The model under review builds one solid part; all positions refer to its coordinate system, in mm. Face numbers are marked on the shaded views. A direction names the side the tool comes from. Coordinates: 2 decimals unless noted, no trailing zeros. Write each loop counter-clockwise with the first axis right and the second up, starting at its lowest first coordinate (ties: lowest second). Pieces come first, ordered by that corner, then holes.
Autodesk Inventor part; units mm, degrees
ref_plane "YZ Plane" through (0, 0, 0) normal (1, 0, 0) x (0, 1, 0)
ref_plane "XZ Plane" through (0, 0, 0) normal (0, 1, 0) x (-1, 0, 0)
ref_plane "XY Plane" through (0, 0, 0) normal (0, 0, 1) x (1, 0, 0)
sketch "Sketch1" plane through (0, 0, 0) normal (0, 1, 0) x (-1, 0, 0)
  arc A0 (52.0258, 55.1946) -> (51.0258, 56.1946) centre (51.0258, 55.1946) ccw
  line L0 (-43.9742, 56.1946) -> (51.0258, 56.1946)
  arc A1 (-43.9742, 56.1946) -> (-44.9742, 55.1946) centre (-43.9742, 55.1946) ccw
  line L1 (-44.9742, -39.8054) -> (-44.9742, 55.1946)
  arc A2 (-44.9742, -39.8054) -> (-43.9742, -40.8054) centre (-43.9742, -39.8054) ccw
  line L2 (51.0258, -40.8054) -> (-43.9742, -40.8054)
  arc A3 (51.0258, -40.8054) -> (52.0258, -39.8054) centre (51.0258, -39.8054) ccw
  line L3 (52.0258, 55.1946) -> (52.0258, -39.8054)
  line L4 (-11.2742, 54.1946) -> (-42.9742, 54.1946)
  line L5 (-11.2742, -38.8054) -> (-11.2742, 54.1946)
  line L6 (-42.9742, -38.8054) -> (-11.2742, -38.8054)
  line L7 (-42.9742, 54.1946) -> (-42.9742, -38.8054)
  line L8 (50.0258, -38.8054) -> (50.0258, 54.1946)
  line L9 (-9.2742, -38.8054) -> (50.0258, -38.8054)
  line L10 (-9.2742, 54.1946) -> (-9.2742, -38.8054)
  line L11 (50.0258, 54.1946) -> (-9.2742, 54.1946)
  line L12 (53.5258, 57.6946) -> (-46.4742, 57.6946)
  line L13 (-46.4742, 57.6946) -> (-46.4742, -42.3054)
  line L14 (-46.4742, -42.3054) -> (53.5258, -42.3054)
  line L15 (53.5258, -42.3054) -> (53.5258, 57.6946)
  line L16 (51.0258, 55.1946) -> (-43.9742, 55.1946) construction
  line L17 (-43.9742, 55.1946) -> (-43.9742, -39.8054) construction
  line L18 (-43.9742, -39.8054) -> (51.0258, -39.8054) construction
  line L19 (51.0258, -39.8054) -> (51.0258, 55.1946) construction
  line L20 (-41.4742, -37.3054) -> (-12.7742, -37.3054)
  line L21 (-12.7742, -37.3054) -> (-12.7742, 52.6946)
  line L22 (-12.7742, 52.6946) -> (-41.4742, 52.6946)
  line L23 (-41.4742, 52.6946) -> (-41.4742, -37.3054)
  line L24 (-7.7742, -37.3054) -> (48.5258, -37.3054)
  line L25 (48.5258, -37.3054) -> (48.5258, 52.6946)
  line L26 (48.5258, 52.6946) -> (-7.7742, 52.6946)
  line L27 (-7.7742, 52.6946) -> (-7.7742, -37.3054)
  line L28 (-10.2742, 55.1946) -> (-10.2742, -39.8054) construction
  arc A4 (51.0258, -40.6054) -> (51.8258, -39.8054) centre (51.0258, -39.8054) ccw
  line L29 (51.0258, -40.6054) -> (-43.9742, -40.6054)
  arc A5 (-44.7742, -39.8054) -> (-43.9742, -40.6054) centre (-43.9742, -39.8054) ccw
  line L30 (-44.7742, -39.8054) -> (-44.7742, 55.1946)
  arc A6 (-43.9742, 55.9946) -> (-44.7742, 55.1946) centre (-43.9742, 55.1946) ccw
  line L31 (-43.9742, 55.9946) -> (51.0258, 55.9946)
  arc A7 (51.8258, 55.1946) -> (51.0258, 55.9946) centre (51.0258, 55.1946) ccw
  line L32 (51.8258, 55.1946) -> (51.8258, -39.8054)
  line L33 (50.2258, 54.3946) -> (50.2258, -39.0054)
  line L34 (50.2258, -39.0054) -> (-9.4742, -39.0054)
  line L35 (-9.4742, -39.0054) -> (-9.4742, 54.3946)
  line L36 (-9.4742, 54.3946) -> (50.2258, 54.3946)
  line L37 (-43.1742, -39.0054) -> (-11.0742, -39.0054)
  line L38 (-11.0742, -39.0054) -> (-11.0742, 54.3946)
  line L39 (-11.0742, 54.3946) -> (-43.1742, 54.3946)
  line L40 (-43.1742, 54.3946) -> (-43.1742, -39.0054)
  point P0 (0, 0)
  point P1 (-29.6242, 39.9946)
  dimension "d0" = 2
  dimension "d1" = 2.5
  dimension "d2" = 2.5
  dimension "d3" = 2.5
  dimension "d4" = 2.5
  dimension "d5" = 2.5
  dimension "d6" = 2.5
  dimension "d7" = 2.5
  dimension "d8" = 2.5
  dimension "d9" = 5
  dimension "d10" = 1
  dimension "d11" = 2
  dimension "d12" = 2.5
  dimension "d13" = 0.2
  dimension "d14" = 0.2
  dimension "d15" = 0.2
extrude "Extrusion1" add sketch "Sketch1" along normal blind 5 contours L3 A3 L2 A2 L1 A1 L0 A0 | L5 L6 L7 L4 | L9 L10 L11 L8 | L15 L14 L13 L12 | L23 L22 L21 L20 | L27 L26 L25 L24 | L29 A5 L30 A6 L31 A7 L32 A4 | L33 L34 L35 L36 | L40 L39 L38 L37
extrude "Extrusion2" add sketch "Sketch1" against normal blind 5 contours L3 A3 L2 A2 L1 A1 L0 A0 | L5 L6 L7 L4 | L9 L10 L11 L8 | L15 L14 L13 L12 | L29 A5 L30 A6 L31 A7 L32 A4 | L33 L34 L35 L36 | L40 L39 L38 L37
extrude "Extrusion3" add sketch "Sketch1" against normal blind 7 contours L29 A5 L30 A6 L31 A7 L32 A4
equation "\"d2\" = d1"
equation "\"d3\" = d2"
equation "\"d4\" = d1"
equation "\"d5\" = d2"
equation "\"d6\" = d1"
equation "\"d7\" = d4"
equation "\"d8\" = d7"
equation "\"d10\" = 0.5 * d11"
equation "\"d12\" = 0.5 * d9"
equation "\"d14\" = d13"
equation "\"d15\" = d14"
properties part number "plantBottomPlate"
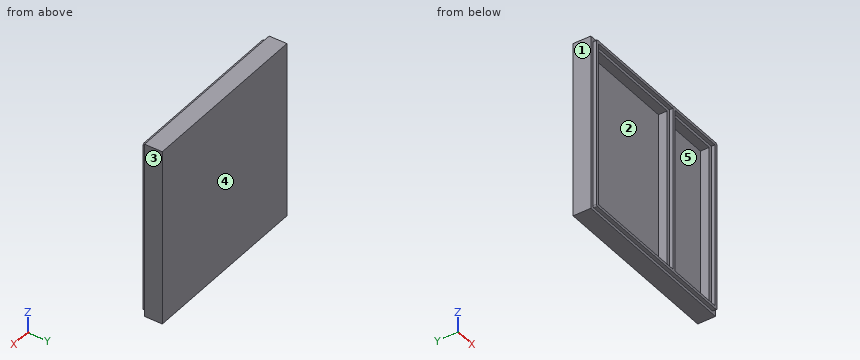
Item 1: Take a section at A-A, the plane x = -47. Write out the cut boundary in (y, z).
Solved:
outline: (-7, -40.61) - (-5, -40.61) - (-5, -42.31) - (5, -42.31) - (5, 57.69) - (-5, 57.69) - (-5, 55.99) - (-7, 55.99) - (-7, 54.39) - (-5, 54.39) - (-5, 52.69) - (0, 52.69) - (0, -37.31) - (-5, -37.31) - (-5, -39.01) - (-7, -39.01) - close
Item 2: For pin 1 (1 mm diameter, centred on x = 6.5, z = 39, fed in from -Y); pin 2 (0.6 mm diameter, centred on x = 20, y = -6.5, fed in from -Z); pin 3 (0.6 mm diameter, centred on y = -6, z = -13, fed in from +X), all flat-tipped, find the tip position at first contact; note any pin that passes through.
Solved:
pin 1: stops at y = 0
pin 2: stops at z = -40.61
pin 3: stops at x = 44.77
Item 3: To check wall thickness, follow line 1 along X through (y, z) = (-0.5, -11); line 2 along X through (y, z) = (-5.5, -31); line 3 along Z through (x, y) = (35, -2). State the ranges of each line that lie inside material, in increasing order.
Solved:
line 1: x = -53.53 to -48.53, 7.77 to 12.77, 41.47 to 46.47
line 2: x = -51.83 to -50.23, 9.47 to 11.07, 43.17 to 44.77
line 3: z = -42.31 to -37.31, 52.69 to 57.69
Item 4: Machinability: for the marked faces 1 and 2, which of the approach directions +Z, -Z, +X, -X, +Y, -Y give a long, thin tool a straight path to every point of the face, cutting with its end or side? Answer none if there is none.
Solved:
face 1: +Z, -Z, -X, +Y, -Y
face 2: -Y
Item 5: Take a section at B-B, the plane z = 20. Write out the cut boundary in (x, y), plus the area to 3 significant figures.
Solved:
outline: (-53.53, -5) - (-51.83, -5) - (-51.83, -7) - (-50.23, -7) - (-50.23, -5) - (-48.53, -5) - (-48.53, 0) - (7.77, 0) - (7.77, -5) - (9.47, -5) - (9.47, -7) - (11.07, -7) - (11.07, -5) - (12.77, -5) - (12.77, 0) - (41.47, 0) - (41.47, -5) - (43.17, -5) - (43.17, -7) - (44.77, -7) - (44.77, -5) - (46.47, -5) - (46.47, 5) - (-53.53, 5) - close
area: 585 mm2
Item 6: Mouldability with a two-part tool opening along X and no side actions: class the marked faces 3, 4 and 5 as pulls with the +X half, pulls with the -X half, needs draft (parallel to the pull), parting line crosses it, or undercut.
Solved:
face 3: pulls with the +X half
face 4: needs draft
face 5: undercut
